from build123d import *

# Parameters (mm, degrees)
F0_W              = 55
F0_H              = 45
F1_DEPTH          = 20
F5_DEPTH          = 17.5
F7_DEPTH          = 2.5
F9_R              = 5
F10_F1_R          = 5
F10_F2_R          = 5
F11_T1_DEPTH      = 35
F11_T3_DEPTH      = 62.5
F11_S7_W          = 5
F11_S7_H          = 5
F11_T8_DEPTH      = 5
F11_T12_ANGLE     = 90
F12_R             = 5
F15_R             = 0.75
F16_DEPTH         = 2.75
F16_COPIES2_COUNT = 2


# Not quite as in the source:
# - a fillet or chamfer that OpenCascade refuses, or shapes differently, is made with other operations: its cross-section is extruded or revolved along the edge and cut away or added
# - a feature of the source that left no trace in its solid (it failed there, or was rolled back) is left out
# - a pattern or mirror of a feature is missing from the dataset's text; its kind, count and spacing are read off the source's solid


with BuildPart() as f1:
    # F0 (on Top) → F1 (new body)
    with BuildSketch(Plane.XY):
        Rectangle(F0_W, F0_H)
    extrude(amount=F1_DEPTH)

    # F4 (on face) → F5 (cut)
    with BuildSketch(Plane.XY.offset(20)):
        with BuildLine():
            Line((-19.5686819828, 11.1526907945), (-19.5686819828, 1.0604560375))
            Line((-19.5686819828, 1.0604560375), (-19.5686819828, -9.0317787194))
            ThreePointArc((-19.5686819828, -9.0317787194), (-17.4612029419, -14.4427117948), (-12.2491327961, -17.0027878582))
            Line((-12.2491327961, -17.0027878582), (-5.4155437946, -17.5861419999))
            ThreePointArc((-5.4155437946, -17.5861419999), (-3.5037525417, -17.5198024128), (-1.6623660017, -17.0014952208))
            Line((-1.6623660017, -17.0014952208), (11.9654898342, -11.3323067543))
            ThreePointArc((11.9654898342, -11.3323067543), (15.5479043196, -8.3854367171), (16.8927628547, -3.9459443945))
            Line((16.8927628547, -3.9459443945), (16.8927628547, 1.0604560375))
            Line((16.8927628547, 1.0604560375), (16.8927628547, 6.0668564696))
            ThreePointArc((16.8927628547, 6.0668564696), (15.5479043196, 10.5063487921), (11.9654898342, 13.4532188293))
            Line((11.9654898342, 13.4532188293), (-1.6623660017, 19.1224072959))
            ThreePointArc((-1.6623660017, 19.1224072959), (-3.5037525417, 19.6407144879), (-5.4155437946, 19.7070540749))
            Line((-5.4155437946, 19.7070540749), (-12.2491327961, 19.1236999333))
            ThreePointArc((-12.2491327961, 19.1236999333), (-17.4612029419, 16.5636238699), (-19.5686819828, 11.1526907945))
        make_face()
    extrude(amount=-F5_DEPTH, mode=Mode.SUBTRACT)

    # F6 (on face) → F7 (join)
    with BuildSketch(Plane.XY.offset(20)):
        with BuildLine():
            ThreePointArc((-12.2491327961, 19.1236999333), (-17.4612029419, 16.5636238699), (-19.5686819828, 11.1526907945))
            Line((-19.5686819828, 11.1526907945), (-19.5686819828, -9.0317787194))
            ThreePointArc((-19.5686819828, -9.0317787194), (-17.4612029419, -14.4427117948), (-12.2491327961, -17.0027878582))
            Line((-12.2491327961, -17.0027878582), (-11.2008683554, -17.0922736911))
            Line((-11.2008683554, -17.0922736911), (-5.4155437946, -17.5861419999))
            ThreePointArc((-5.4155437946, -17.5861419999), (-3.5037525417, -17.5198024128), (-1.6623660017, -17.0014952208))
            Line((-1.6623660017, -17.0014952208), (11.9654898342, -11.3323067543))
            ThreePointArc((11.9654898342, -11.3323067543), (15.5479043196, -8.3854367171), (16.8927628547, -3.9459443945))
            Line((16.8927628547, -3.9459443945), (16.8927628547, 6.0668564696))
            ThreePointArc((16.8927628547, 6.0668564696), (15.5479043196, 10.5063487921), (11.9654898342, 13.4532188293))
            Line((11.9654898342, 13.4532188293), (-1.6432446132, 19.1144527977))
            Line((-1.6432446132, 19.1144527977), (-1.6623660017, 19.1224072959))
            ThreePointArc((-1.6623660017, 19.1224072959), (-3.5037525417, 19.6407144879), (-5.4155437946, 19.7070540749))
            Line((-5.4155437946, 19.7070540749), (-12.2491327961, 19.1236999333))
        make_face()
        with BuildLine():
            Line((-12.2647350556, -9.6505587512), (-12.2647350556, 0.4416760057))
            Line((-12.2647350556, 0.4416760057), (-12.2647350556, 10.5339107627))
            ThreePointArc((-12.2647350556, 10.5339107627), (-11.0828219735, 13.1216791931), (-8.6049604623, 14.5194153321))
            Line((-8.6049604623, 14.5194153321), (-1.7713714607, 15.1027694737))
            ThreePointArc((-1.7713714607, 15.1027694737), (-0.8154758343, 15.0695996802), (0.1052174357, 14.8104460842))
            Line((0.1052174357, 14.8104460842), (13.7330732716, 9.1412576176))
            ThreePointArc((13.7330732716, 9.1412576176), (15.4399139751, 7.6115436145), (16.1967097819, 5.4480764378))
            Line((16.1967097819, 5.4480764378), (16.1967097819, 0.4416760057))
            Line((16.1967097819, 0.4416760057), (16.1967097819, -4.5647244263))
            ThreePointArc((16.1967097819, -4.5647244263), (15.5242805143, -6.7844705876), (13.7330732716, -8.2579056062))
            Line((13.7330732716, -8.2579056062), (0.1052174357, -13.9270940728))
            ThreePointArc((0.1052174357, -13.9270940728), (-0.8154758343, -14.1862476688), (-1.7713714607, -14.2194174623))
            Line((-1.7713714607, -14.2194174623), (-8.6049604623, -13.6360633206))
            ThreePointArc((-8.6049604623, -13.6360633206), (-11.2109955351, -12.3560252889), (-12.2647350556, -9.6505587512))
        make_face(mode=Mode.SUBTRACT)
    extrude(amount=-F7_DEPTH)

    # F9
    f9_edges = [f1.edges().sort_by_distance(p)[0] for p in [
        (-27.5, -22.5, 10),
        (0, -22.5, 20),
    ]]
    fillet(f9_edges, radius=F9_R)

    # F10: fillet of radius 5 on 2 edges, made by hand

    # F10_f1
    f10_f1_edges = [f1.edges().sort_by_distance(p)[0] for p in [
        (0, 22.5, 0),
    ]]
    fillet(f10_f1_edges, radius=F10_F1_R)

    # F10_f2
    f10_f2_edges = [f1.edges().sort_by_distance(p)[0] for p in [
        (-27.5, 22.5, 12.5),
    ]]
    fillet(f10_f2_edges, radius=F10_F2_R)

    # F11: fillet of radius 5 on 2 edges, made by hand

    # F11_s2 → F11_t1 (cut)
    with BuildSketch(Plane.XZ.offset(-17.5)):
        with BuildLine():
            ThreePointArc((-22.5, 20), (-26.0355339059, 18.5355339059), (-27.5, 15))
            Line((-27.5, 15), (-27.5, 20))
            Line((-27.5, 20), (-22.5, 20))
        make_face()
    extrude(amount=F11_T1_DEPTH, mode=Mode.SUBTRACT)

    # F11_s4 → F11_t3 (cut)
    with BuildSketch(Plane.YZ.offset(-22.5)):
        with BuildLine():
            ThreePointArc((22.5, 15), (21.0355339059, 18.5355339059), (17.5, 20))
            Line((17.5, 20), (22.5, 20))
            Line((22.5, 20), (22.5, 15))
        make_face()
    extrude(amount=F11_T3_DEPTH, mode=Mode.SUBTRACT)


with BuildPart() as f11_tool6:
    # F11_s7 → F11_t8 (new body)
    with BuildSketch(Plane.XY.offset(15)):
        with Locations((-25, -20)):
            Rectangle(F11_S7_W, F11_S7_H)
    extrude(amount=F11_T8_DEPTH)

    # F11_s9 → F11_t10 (revolve, cut)
    with BuildSketch(Plane(origin=(-22.5, -17.5, 15), x_dir=(0.7071067812, 0.7071067812, 0), z_dir=(0.7071067812, -0.7071067812, 0))):
        with BuildLine():
            ThreePointArc((0, -5), (5, 0), (0, 5))
            Line((0, 5), (0, -5))
        make_face()
    revolve(axis=Axis((-22.5, -17.5, 15), (0, 0, 1)), mode=Mode.SUBTRACT)


with BuildPart() as f1_1:
    add(f1.part)

    # F11_t5: cut F11_tool6
    add(f11_tool6.part, mode=Mode.SUBTRACT)

    # F11_s11 → F11_t12 (revolve, cut)
    with BuildSketch(Plane.YZ.offset(-22.5)):
        with BuildLine():
            ThreePointArc((17.5, 20), (21.0355339059, 18.5355339059), (22.5, 15))
            Line((22.5, 15), (22.5, 20))
            Line((22.5, 20), (17.5, 20))
        make_face()
    revolve(axis=Axis((-22.5, 17.5, 20), (0, 0, 1)), revolution_arc=F11_T12_ANGLE, mode=Mode.SUBTRACT)

    # F12
    f12_edges = [f1_1.edges().sort_by_distance(p)[0] for p in [
        (-22.5, -22.5, 10),
        (27.5, 21.035534, 1.464466),
        (27.5, 22.5, 10),
        (27.5, 21.035534, 18.535534),
        (27.5, 0, 20),
        (27.5, -21.035534, 18.535534),
        (27.5, -22.5, 10),
        (27.5, -21.035534, 1.464466),
    ]]
    fillet(f12_edges, radius=F12_R)

    # F15 (on offset) → F16 (join)
    with BuildSketch(Plane.XZ.offset(12.75)):
        with BuildLine():
            Line((30.0576982113, 5), (27.5, 5))
            ThreePointArc((27.5, 5), (26.0355339059, 1.4644660941), (22.5, 0))
            Line((22.5, 0), (32.8350702046, 0))
            Line((32.8350702046, 0), (32.8350702046, 2.5))
            ThreePointArc((32.8350702046, 2.5), (32.2693847797, 2.7343145751), (32.0350702046, 3.3))
            ThreePointArc((32.0350702046, 3.3), (31.3615386923, 4.5165750888), (30.0576982113, 5))
        make_face()
        with Locations((30.0576982113, 3)):
            Circle(F15_R, mode=Mode.SUBTRACT)
    f16 = extrude(amount=-F16_DEPTH)

    # F16_copies: F16 across plane
    add(f16.mirror(Plane(origin=(0, 0, 0), x_dir=(0, 0, -1), z_dir=(-1, 0, 0))))

    # F16_copies1: F16 across plane
    add(f16.mirror(Plane.ZX))

    # F16_copies2: F16 ×2 about axis
    f16_copies2_axis = Axis((0, 0, 0), (0, 0, 1))
    for i in range(1, F16_COPIES2_COUNT):
        add(f16.rotate(f16_copies2_axis, i * 360 / F16_COPIES2_COUNT))


solid = f1_1.part
Read the model definition and answer for the solid it produces. Units are mm, in the model's axes. A direction names the side the tool comes from. Coordinates: 2 decimals unless noted, no trailing zeros. Write each loop counter-clockwise with the first axis right and the second up, starting at its lowest first coordinate (ties: lowest second). Pieces come first, ordered by that corner, then holes. Notation, with made-up numbers: (52, 2) -> (104, 2) arc R23 cw to (104, 37) -> close; hole circle Ø1 at (59, 65). An arc over 180 degrees is marked (long way). Return JSON: item names as keys, results as strings.
(1) The part is cut by section D-D on z = 18.5. Give the vertices of the cut face in (x, y), then the cut area to 3 significant figures.
Answers below:
{"outline": "(-26.07, -17.5) arc R3.57 ccw to (-22.5, -21.07) -> (22.5, -21.07) arc R3.57 ccw to (26.07, -17.5) -> (26.07, 17.5) arc R3.57 ccw to (22.5, 21.07) -> (-22.5, 21.07) arc R3.57 ccw to (-26.07, 17.5) -> close; hole (-12.26, -9.65) arc R4 ccw to (-8.6, -13.64) -> (-1.77, -14.22) arc R4 ccw to (0.11, -13.93) -> (13.73, -8.26) arc R4 ccw to (16.2, -4.56) -> (16.2, 5.45) arc R4.6 ccw to (13.73, 9.14) -> (0.11, 14.81) arc R4 ccw to (-1.77, 15.1) -> (-8.6, 14.52) arc R4.6 ccw to (-12.26, 10.53) -> close", "area": "1,490 mm^2"}
(2) Consider line 1 along Z through (x, y) = (8, -12.5); line 2 along Y through (x, z) = (13.5, 18); line 3 along X through (y, z) = (-8, 4.5). Determine where each line is inside the solid, lowest interval first. Write a range as from..to.
Answers below:
{"line 1": "0..2.5, 17.5..20", "line 2": "-21.5..-8.35, 9.24..21.5", "line 3": "-27.47..-19.57, 15.79..27.47"}
(3) The part is cut by section C-C on x = 5.5. Give the vertices of the cut face in (y, z), then the cut area to 3 significant figures.
Answers below:
{"outline": "(-22.5, 5) arc R5 ccw to (-17.5, 0) -> (17.5, 0) arc R5 ccw to (22.5, 5) -> (22.5, 15) arc R5 ccw to (17.5, 20) -> (12.57, 20) -> (12.57, 17.5) -> (16.14, 17.5) -> (16.14, 2.5) -> (-14.02, 2.5) -> (-14.02, 17.5) -> (-11.68, 17.5) -> (-11.68, 20) -> (-17.5, 20) arc R5 ccw to (-22.5, 15) -> close", "area": "365 mm^2"}
(4) Which of the six approach directions +Z, -Z, +X, -X, +Y, -Y give full straight-line access (tool end or side, diameter ignored) to faces 4 (the flat face through (16.197, 1, 19)), 5 (the flat face through (16.893, 1, 10)), 6 (the cylindrical face through (26, -15.16, 1.43)), 7 (the cylindrical face through (-26.07, 15.16, 1.5))?
Answers below:
{"face 4": "+Z", "face 5": "none", "face 6": "-Z, +X, -Y", "face 7": "-Z, -X, +Y"}
(5) For a pull along Z with two mould halves and no side action, classify faces 1 (the flat face through (29, 11, 5)), 2 (the flat face through (0, -22.5, 10)), 3 (the flat face through (5.247, 16.248, 10.105)) as pulls with the +Z half, pulls with the -Z half, needs draft (parallel to the pull), parting line crosses it, or undercut.
Answers below:
{"face 1": "pulls with the +Z half", "face 2": "needs draft", "face 3": "undercut"}
(6) The part is cut by section A-A on z = 6. Give the vertices of the cut face in (x, y), then the cut area to 3 significant figures.
Answers below:
{"outline": "(-27.5, -17.5) arc R5 ccw to (-22.5, -22.5) -> (22.5, -22.5) arc R5 ccw to (27.5, -17.5) -> (27.5, 17.5) arc R5 ccw to (22.5, 22.5) -> (-22.5, 22.5) arc R5 ccw to (-27.5, 17.5) -> close; hole (-19.57, -9.03) arc R8 ccw to (-12.25, -17) -> (-5.42, -17.59) arc R8 ccw to (-1.66, -17) -> (11.97, -11.33) arc R8 ccw to (16.89, -3.95) -> (16.89, 6.07) arc R8 ccw to (11.97, 13.45) -> (-1.66, 19.12) arc R8 ccw to (-5.42, 19.71) -> (-12.25, 19.12) arc R8 ccw to (-19.57, 11.15) -> close", "area": "1,310 mm^2"}
(7) Each of these flat-tipped pins is pushed along its axis until it touches: P1, Ø18, axis at x = -2.5, y = 1, coming from the +Z side; P2, Ø12, axis at y = -15, z = 11, coming from the +X side; P3, Ø0.8, axis at y = -0.5, z = 19, coming from the +X side; P4, Ø0.9, axis at x = -30.06, z = 3, coming from the -Y side. Where does it stop, or does it pass through?
Answers below:
{"P1": "z = 2.5", "P2": "x = 27.5", "P3": "x = 25.97", "P4": "through"}
(8) The part is cut by section B-B on y = 12. Give the vertices of the cut face in (x, z), then the cut area to 3 significant figures.
Answers below:
{"outline": "(-32.84, 0) -> (32.84, 0) -> (32.84, 2.5) arc R0.8 cw to (32.04, 3.3) arc R2 ccw to (30.06, 5) -> (27.5, 5) -> (27.5, 15) arc R5 ccw to (22.5, 20) -> (6.86, 20) -> (6.86, 17.5) -> (14.26, 17.5) -> (14.26, 2.5) -> (-19.52, 2.5) -> (-19.52, 17.5) -> (-11.84, 17.5) -> (-11.84, 20) -> (-22.5, 20) arc R5 ccw to (-27.5, 15) -> (-27.5, 5) -> (-30.06, 5) arc R2 ccw to (-32.04, 3.3) arc R0.8 cw to (-32.84, 2.5) -> close; hole circle Ø1.5 at (-30.06, 3); hole circle Ø1.5 at (30.06, 3)", "area": "580 mm^2"}
